```python
from build123d import *

# Parameters (mm, degrees)
BOSS_EXTRUDE1_DEPTH   = 22
FILLET1_R             = 2
F_3_0MM_DOWEL_HOLE2_D = 3
CONVERT_SOLID1_DEPTH  = 22
M3_CLEARANCE_HOLE1_D  = 3.4


# Read off the part's stored shape, not the designer's step: Convert-Solid1
with BuildPart() as part:
    # Sketch1 → Boss-Extrude1 (new body)
    with BuildSketch(Plane(origin=(0, 0, 0), x_dir=(0, 0, -1), z_dir=(1, 0, 0))):
        with BuildLine():
            Line((-45, -15), (-37.195759655, -19.505780264))
            ThreePointArc((-37.195759655, -19.505780264), (-24.9972884, -33.75108254), (-7.814503261, -41.266615306))
            Line((-7.814503261, -41.266615306), (7.814503261, -41.266615306))
            ThreePointArc((7.814503261, -41.266615306), (24.9972884, -33.75108254), (37.195759655, -19.505780264))
            Line((37.195759655, -19.505780264), (45, -15))
            Line((45, -15), (45, 0))
            Line((45, 0), (47, 0))
            Line((47, 0), (47, -16.154700538))
            Line((47, -16.154700538), (38.691455747, -20.9516408))
            ThreePointArc((38.691455747, -20.9516408), (25.874940227, -35.587743231), (8, -43.266615306))
            Line((8, -43.266615306), (-8, -43.266615306))
            ThreePointArc((-8, -43.266615306), (-25.874940227, -35.587743231), (-38.691455747, -20.9516408))
            Line((-38.691455747, -20.9516408), (-47, -16.154700538))
            Line((-47, -16.154700538), (-47, 0))
            Line((-47, 0), (-45, 0))
            Line((-45, 0), (-45, -15))
        make_face()
    extrude(amount=BOSS_EXTRUDE1_DEPTH)

    # Fillet1
    fillet1_edges = [part.edges().sort_by_distance(p)[0] for p in [
        (11, -16.154700538, 47),
        (11, -15, 45),
        (11, -19.505780264, 37.195759655),
        (11, -41.266615306, 7.814503261),
        (11, -41.266615306, -7.814503261),
        (11, -19.505780264, -37.195759655),
        (11, -15, -45),
        (11, -16.154700538, -47),
        (11, -20.9516408, -38.691455747),
        (11, -43.266615306, -8),
        (11, -43.266615306, 8),
        (11, -20.9516408, 38.691455747),
    ]]
    fillet(fillet1_edges, radius=FILLET1_R)

    # Ø3.0mm Dowel Hole2 (through all)
    with Locations(Plane.XY.offset(47)):
        with Locations((4, -10), (12, -10), (12, -4)):
            Hole(F_3_0MM_DOWEL_HOLE2_D / 2)

    # Convert-Solid1 outline → Convert-Solid1 (cut)
    with BuildSketch(Plane.YZ):
        with BuildLine():
            ThreePointArc((-13.845299462, -47), (-15.845299462, -46.464101615), (-17.309401077, -45))
            Line((-17.309401077, -45), (-16.732050808, -46))
            ThreePointArc((-16.732050808, -46), (-16, -46.732050808), (-15, -47))
            Line((-15, -47), (-13.845299462, -47))
        make_face()
        with BuildLine():
            Line((-16.732050808, 46), (-17.309401077, 45))
            ThreePointArc((-17.309401077, 45), (-15.845299462, 46.464101615), (-13.845299462, 47))
            Line((-13.845299462, 47), (-15, 47))
            ThreePointArc((-15, 47), (-16, 46.732050808), (-16.732050808, 46))
        make_face()
        with BuildLine():
            ThreePointArc((-20.672392382, 39.175128193), (-21.000794949, 38.750427658), (-21.430336964, 38.428383489))
            ThreePointArc((-21.430336964, 38.428383489), (-21.191397112, 38.560662449), (-20.9516408, 38.691455747))
            Line((-20.9516408, 38.691455747), (-20.672392382, 39.175128193))
        make_face()
        with BuildLine():
            Line((-43.266615306, 7.814503261), (-43.266615306, 7.624494898))
            ThreePointArc((-43.266615306, 7.624494898), (-43.248238475, 8.007479152), (-43.193276836, 8.386944387))
            ThreePointArc((-43.193276836, 8.386944387), (-43.212600611, 8.286805686), (-43.231692225, 8.186622464))
            ThreePointArc((-43.231692225, 8.186622464), (-43.257865395, 8.001380442), (-43.266615306, 7.814503261))
        make_face()
        with BuildLine():
            ThreePointArc((-43.231692225, -8.186622464), (-43.212600611, -8.286805686), (-43.193276836, -8.386944387))
            ThreePointArc((-43.193276836, -8.386944387), (-43.248238475, -8.007479152), (-43.266615306, -7.624494898))
            Line((-43.266615306, -7.624494898), (-43.266615306, -7.814503261))
            ThreePointArc((-43.266615306, -7.814503261), (-43.257865395, -8.001380442), (-43.231692225, -8.186622464))
        make_face()
        with BuildLine():
            ThreePointArc((-21.430336964, -38.428383489), (-21.000794949, -38.750427658), (-20.672392382, -39.175128193))
            Line((-20.672392382, -39.175128193), (-20.9516408, -38.691455747))
            ThreePointArc((-20.9516408, -38.691455747), (-21.191397112, -38.560662449), (-21.430336964, -38.428383489))
        make_face()
    extrude(amount=CONVERT_SOLID1_DEPTH, mode=Mode.SUBTRACT)

    # M3 Clearance Hole1 (through all)
    with Locations(Plane(origin=(0, -41.266615306, 0), x_dir=(1, 0, 0), z_dir=(0, 1, 0))):
        with Locations((10, 3.99745139), (10, -4.00254861)):
            Hole(M3_CLEARANCE_HOLE1_D / 2)


solid = part.part
```
Geometry: final body of the model. Coordinates: model frame, mm. A direction names the side the tool comes from. Round coordinates to 2 decimals unless told otherwise and drop trailing zeros. Write each loop counter-clockwise with the first axis right and the second up, starting at its lowest first coordinate (ties: lowest second). Pieces come first, ordered by that corner, then holes. Notation, with made-up numbers: (34.5, 63.25) -> (68.5, 63.25) arc R9 ccw to (68.5, 73.25) -> close; hole circle Ø8 at (61.5, 11.5). An arc over 180 degrees is marked (long way). Return JSON: item names as keys, results as strings.
Q1. Section A-A on x = 14.5. Return the cut outline in (y, z), and give its area (3 significant figures).
From the geometry:
{"outline": "(-43.27, -7.62) arc R4 ccw to (-43.19, -8.39) arc R44 ccw to (-21.43, -38.43) arc R44 ccw to (-20.95, -38.69) -> (-17.31, -45) arc R4 ccw to (-13.85, -47) -> (0, -47) -> (0, -45) -> (-13.85, -45) arc R2 cw to (-15.58, -44) -> (-19.22, -37.69) arc R2 ccw to (-20, -36.93) arc R42 cw to (-41.23, -8.01) arc R2 cw to (-41.27, -7.62) -> (-41.27, 7.62) arc R2 cw to (-41.23, 8.01) arc R42 cw to (-20, 36.93) arc R2 ccw to (-19.22, 37.69) -> (-15.58, 44) arc R2 cw to (-13.85, 45) -> (0, 45) -> (0, 47) -> (-13.85, 47) arc R4 ccw to (-17.31, 45) -> (-20.95, 38.69) arc R44 ccw to (-21.43, 38.43) arc R44 ccw to (-43.19, 8.39) arc R4 ccw to (-43.27, 7.62) -> close", "area": "284 mm2"}
Q2. Section C-C on z = 31. Return the cut outline in (x, y), and give its area (3 significant figures).
From the geometry:
{"outline": "(0, -31.22) -> (22, -31.22) -> (22, -28.34) -> (0, -28.34) -> close", "area": "63.5 mm2"}
Q3. Section B-B on y = -24. Return the cut outline in (x, z), and give its area (3 significant figures).
From the geometry:
{"outline": "(0, -36.88) -> (22, -36.88) -> (22, -34.47) -> (0, -34.47) -> close; (0, 34.47) -> (22, 34.47) -> (22, 36.88) -> (0, 36.88) -> close", "area": "106 mm2"}
Q4. Ray query, line 1 (Y direction, x = 12, z = 45.6); line 2 (Z direction, x = 18.5, y = -2); line 3 (Y direction, x = 12, z = 46.2). Return the intervals inside material, ascending.
From the geometry:
{"line 1": "-16.89 to -11.5, -8.5 to -5.5, -2.5 to 0", "line 2": "-47 to -45, 45 to 47", "line 3": "-16.25 to -11.5, -8.5 to -5.5, -2.5 to 0"}
Q5. Set-up query: faces 5 (the flat face through (10.846, -17.424, -40.802)), 6 (the cylindrical face through (4.325, -11.464, -46.014)). Return all of +Z, -Z, +X, -X, +Y, -Y with unobstructed straight access to the full face (end or side cutting, diameter ignored); none if empty.
From the geometry:
{"face 5": "+X, -X, +Y", "face 6": "+Z, -Z"}
Q6. First-contact query: pin 1 Ø10 at (x, z) = (6.5, -18) entering from +Y; pin 2 Ø12 at (x, z) = (9, 4) entering from +Y; pin 3 Ø5 at (x, y) = (15.5, -35) entering from +Z. Flat tips, straight axial feed; report the tip coordinate or a pass-through.
From the geometry:
{"pin 1": "y = -35.14", "pin 2": "y = -40.79", "pin 3": "z = 29.66"}
Q7. Section D-D on z = -19. Return the cut outline in (x, y).
From the geometry:
{"outline": "(0, -39.69) -> (22, -39.69) -> (22, -37.46) -> (0, -37.46) -> close"}
Q8. Mould query, pull axis Y, two halves, no side actions, for faces 1 (the flat face through (11, -7, 47)), 2 (the cylindrical face through (13.2, -10.9, 46)), 3 (the cylindrical face through (10.846, -35.789, 25.596)), 4 (the flat face through (11, 0, 46)). Classes: +Y half, -Y half, draft (parallel to the pull), parting line (faces both ways), or undercut.
From the geometry:
{"face 1": "draft", "face 2": "undercut", "face 3": "-Y half", "face 4": "+Y half"}
